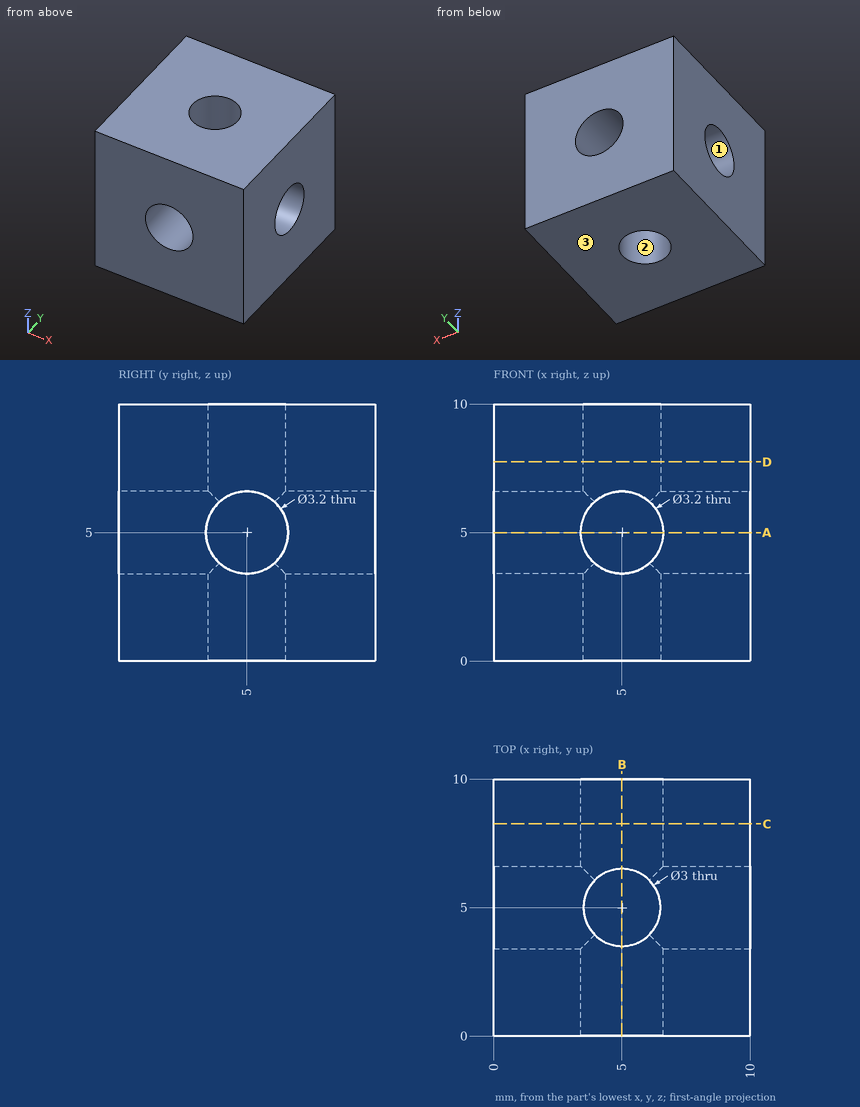
Geometry: see drawing. Coordinates: mm, zero at the bounding-box minimum. Round coordinates to 2 decimals unless told otherwise and drop trailing zeros. Loops run counter-clockwise (first coordinate to the right, second up) from the corner with the lowest first, then second, coordinate; pieces in that order, holes last. Notation, with made-up numbers: (-16, 75.25) -> (16, 75.25) arc R28 cw to (16, 94.25) -> close; hole circle Ø5 at (37, 18.5). An arc over 180 degrees is marked (long way). One line per question, with ' | ' between items. Start each with the question number.
1. Line query: line 1 along Y through (x, z) = (8, 5); line 2 along Y through (x, z) = (5, 2.15). Output: solid intervals per line, ascending. Write a range as [from, to].
2. Section C-C on y = 8.25. Output: boundary loops of the cut face in (x, z).
3. Section B-B on x = 5. Output: boundary loops of the cut face in (y, z), and give its area (3 significant figures).
4. Section A-A on z = 5. Output: boundary loops of the cut face in (x, y), and give its area (3 significant figures).
5. Section D-D on z = 7.75. Output: boundary loops of the cut face in (x, y).
6. Mould query, pull axis Z, two halves, no side actions, for the marked faces 1, 2 and 3. Classes: pulls with the +Z half, pulls with the -Z half, needs draft (parallel to the pull), parting line crosses it, or undercut.
Returned:
1) line 1: y = [0, 3.4], [6.6, 10] | line 2: y = [0, 3.5], [6.5, 10]
2) outline: (0, 0) -> (10, 0) -> (10, 10) -> (0, 10) -> close; hole circle Ø3.2 at (5, 5)
3) outline: (0, 0) -> (3.5, 0) -> (3.5, 3.4) -> (0, 3.4) -> close; (0, 6.6) -> (3.5, 6.6) -> (3.5, 10) -> (0, 10) -> close; (6.5, 0) -> (10, 0) -> (10, 3.4) -> (6.5, 3.4) -> close; (6.5, 6.6) -> (10, 6.6) -> (10, 10) -> (6.5, 10) -> close | area: 47.6 mm2
4) outline: (0, 0) -> (3.4, 0) -> (3.4, 3.4) -> (0, 3.4) -> close; (0, 6.6) -> (3.4, 6.6) -> (3.4, 10) -> (0, 10) -> close; (6.6, 0) -> (10, 0) -> (10, 3.4) -> (6.6, 3.4) -> close; (6.6, 6.6) -> (10, 6.6) -> (10, 10) -> (6.6, 10) -> close | area: 46.2 mm2
5) outline: (0, 0) -> (10, 0) -> (10, 10) -> (0, 10) -> close; hole circle Ø3 at (5, 5)
6) face 1: undercut | face 2: needs draft | face 3: pulls with the -Z half
